Here's the drawing with two shaded views (mm, measured from the low corner). I have some questions. Round coordinates to 2 decimals unless told otherwise and drop trailing zeros. Loops run counter-clockwise (first coordinate to the right, second up) from the corner with the lowest first, then second, coordinate; pieces in that order, holes last. Notation, with made-up numbers: (-29, 9) - (14, 9) arc R17 cw to (14, 42) - close; hole circle Ø3 at (32.5, 50.5). An arc over 180 degrees is marked (long way). Use one line per item in the form item = value.
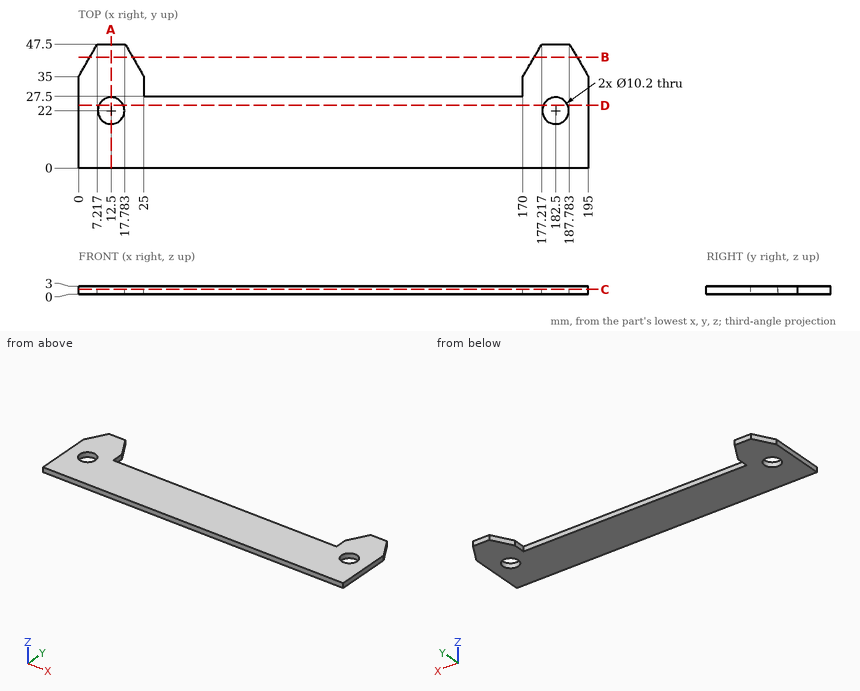
1. If we section it at B-B, the plane y = 42.5: Write out the boundary of the cut face in (x, z).
Solution:
outline = (4.33, 0) - (20.67, 0) - (20.67, 3) - (4.33, 3) - close; (174.33, 0) - (190.67, 0) - (190.67, 3) - (174.33, 3) - close
2. If we section it at A-A, the plane x = 12.5: Write out the boundary of the cut face in (y, z), plus the area to 3 significant figures.
Solution:
outline = (0, 0) - (16.9, 0) - (16.9, 3) - (0, 3) - close; (27.1, 0) - (47.5, 0) - (47.5, 3) - (27.1, 3) - close
area = 112 mm^2
3. If we section it at D-D, the plane y = 24: Write out the boundary of the cut face in (x, z), plus the area to 3 significant figures.
Solution:
outline = (0, 0) - (7.81, 0) - (7.81, 3) - (0, 3) - close; (17.19, 0) - (177.81, 0) - (177.81, 3) - (17.19, 3) - close; (187.19, 0) - (195, 0) - (195, 3) - (187.19, 3) - close
area = 529 mm^2
4. If we section it at C-C, the plane z = 1.8: Write out the boundary of the cut face in (x, y), plus the area to 3 significant figures.
Solution:
outline = (0, 0) - (195, 0) - (195, 35) - (187.78, 47.5) - (177.22, 47.5) - (170, 35) - (170, 27.5) - (25, 27.5) - (25, 35) - (17.78, 47.5) - (7.22, 47.5) - (0, 35) - close; hole circle Ø10.2 at (12.5, 22); hole circle Ø10.2 at (182.5, 22)
area = 6,020 mm^2
5. For P1, Ø1.5, axis at x = 113.5, z = 2, coming from the +Y side, with a flat end and sliding along its axis, tell me the tip position at first contact or that it passes through.
Solution:
P1 = 27.5
6. Please list where these lines run through material, in increasing order: line 1 along Y through (x, z) = (12.5, 1.05); line 2 along X through (y, z) = (24, 1.75); line 3 along Y through (x, z) = (112.5, 0.4).
Solution:
line_1 = 0 to 16.9, 27.1 to 47.5
line_2 = 0 to 7.81, 17.19 to 177.81, 187.19 to 195
line_3 = 0 to 27.5
